```python
from build123d import *

# Parameters (mm, degrees)
SKETCH2_R            = 13.125
F_26_25_MM_HUL_DEPTH = 50
CUT_EXTRUDE1_DEPTH   = 50


with BuildPart() as part:
    # Sketch1 → Base-Revolve (revolve)
    with BuildSketch(Plane.XY):
        with BuildLine():
            Line((28, 0), (28, 39.6))
            ThreePointArc((28, 39.6), (27.882842712, 39.882842712), (27.6, 40))
            Line((27.6, 40), (-74.690598923, 40))
            Line((-74.690598923, 40), (-77, 36))
            Line((-77, 36), (-80, 36))
            Line((-80, 36), (-80, 34.9))
            ThreePointArc((-80, 34.9), (-80.191000574, 34.558943934), (-80.5815962, 34.54359739))
            Line((-80.5815962, 34.54359739), (-81.477336756, 35))
            Line((-81.477336756, 35), (-83.6, 35))
            ThreePointArc((-83.6, 35), (-83.882842712, 34.882842712), (-84, 34.6))
            Line((-84, 34.6), (-84, 25))
            Line((-84, 25), (-47, 25))
            Line((-47, 25), (-32.56624327, 0))
            Line((-32.56624327, 0), (28, 0))
        make_face()
    revolve(axis=Axis((-90.573458716, 0, 0), (1, 0, 0)))

    # Sketch2 → ø26.25 mm hul (cut, symmetric)
    with BuildSketch(Plane.XY):
        Circle(SKETCH2_R)
    extrude(amount=F_26_25_MM_HUL_DEPTH, both=True, mode=Mode.SUBTRACT)

    # Sketch3 → Cut-Extrude1 (cut, symmetric)
    with BuildSketch(Plane(origin=(0, 0, 0), x_dir=(1, 0, 0), z_dir=(0, 1, 0))):
        with BuildLine():
            Line((28, 25), (-39, 25))
            ThreePointArc((-39, 25), (-39.707106781, 25.292893219), (-40, 26))
            Line((-40, 26), (-40, 40))
            Line((-40, 40), (28, 40))
            Line((28, 40), (28, 25))
        make_face()
        with BuildLine():
            Line((-40, -26), (-40, -40))
            Line((-40, -40), (28, -40))
            Line((28, -40), (28, -25))
            Line((28, -25), (-39, -25))
            ThreePointArc((-39, -25), (-39.707106781, -25.292893219), (-40, -26))
        make_face()
    extrude(amount=CUT_EXTRUDE1_DEPTH, both=True, mode=Mode.SUBTRACT)

    # Sketch4 → Cut-Revolve1 (revolve, cut)
    with BuildSketch(Plane.XY):
        Polygon((28, -9.5), (27, -9.5), (27, -14), (8, -14), (6.267949192, -17), (-52, -17), (-55.75277675, -23.5), (28, -23.5), align=None)
    revolve(axis=Axis((28, -23.5, 0), (-1, 0, 0)), mode=Mode.SUBTRACT)


solid = part.part
```
Geometry check sheet. Reference: the model listing, model coordinates, mm. A direction names the side the tool comes from. Give positions to 0.01 mm unless a question says otherwise; leave off trailing zeros. Order: outer loops, then holes, each group sorted by start corner. A loop starts at its lowest first (then second) coordinate and runs counter-clockwise, first axis right, second up. Notation, with made-up numbers: (0, 20) - (15, 20) arc R12 ccw to (15, 31) - close; hole circle Ø6 at (-11.5, -27.75). An arc over 180 degrees is marked (long way). Write item = value, one per line. Start each with the question number.
1) Section check D-D (x = 17). Enter the section's corners in (y, z).
2) Gauge pin test, flat ends, axial feed: pin 1 Ø17 at (y, z) = (-23.5, 0) entering from +X; pin 2 Ø5 at (x, y) = (3.5, -12) entering from -Z; pin 3 Ø10 at (x, z) = (-7, 27.5) entering from -Y. Record the tip position at first contact, or that the pin passes through.
3) Access from +Z, -Z, +X, -X, +Y, -Y to the whole of each face (thin tool, end or side, straight path). Record for faces 1 (the flat face through (-12, 7, 25)), 2 (the cylindrical face through (-65.241, 23.846, 7.509)), 3 (the flat face through (28, 9, 0)), 4 (the conical face through (-53.79, -26.9, -0.07)), 5 (the flat face through (-84, 22.9, 10.4)).
4) Section check B-B (x = -23). Enter the section's corners in (y, z).
5) Section check A-A (x = 0). Enter the section's corners in (y, z) (3 decimals), then the cut area to 3 significant figures.
6) Scan lines: L1, parallel to Z at x = 18.25, y = -23.5; L2, parallel to Y at x = -43.5, z = 5.5; L3, parallel to Z at x = 27.5, y = -23.5. Record each from-to range of solid material in increasing order.
7) Draft check along Y on faces 6 (the cylindrical face through (-35.63, 36.95, -15.32)), 7 (the flat face through (-40, 0, -31)), 8 (the conical face through (-34.871, 3.807, 1.199)). Enter one of: released by +Y, released by -Y, zero draft, split by the parting line, or undercut.
8) Section check C-C (x = -36.5). Enter the section's corners in (y, z), then the cut area to 3 significant figures.
Geometry check:
q1.outline = (-31.22, -25) - (31.22, -25) arc R40 ccw to (31.22, 25) - (-31.22, 25) arc R40 ccw to start; hole circle Ø19 at (-23.5, 0)
q2.pin_1 = 7.42
q2.pin_2 = -25
q2.pin_3 = -33.07
q3.face_1 = +Z, +X, +Y, -Y
q3.face_2 = -X
q3.face_3 = +Z, -Z, +X, +Y, -Y
q3.face_4 = +X
q3.face_5 = +Z, -Z, -X, +Y, -Y
q4.outline = (-31.22, -25) - (31.22, -25) arc R40 ccw to (31.22, 25) - (-31.22, 25) arc R40 ccw to start; hole circle Ø13 at (-23.5, 0)
q5.outline = (-31.225, -25) - (-13.125, -25) - (-13.125, 25) - (-31.225, 25) arc R40 ccw to start; (13.125, -25) - (31.225, -25) arc R40 ccw to (31.225, 25) - (13.125, 25) - close; hole circle Ø13 at (-23.5, 0)
q5.area = 2,280 mm2
q6.L1 = -25 to -9.5, 9.5 to 25
q6.L2 = -39.62 to -26.96, -20.04 to -18.12, 18.12 to 39.62
q6.L3 = -25 to -14, 14 to 25
q7.face_6 = split by the parting line
q7.face_7 = zero draft
q7.face_8 = undercut
q8.outline = (-31.22, -25) - (31.22, -25) arc R40 ccw to (31.22, 25) - (-31.22, 25) arc R40 ccw to start; hole circle Ø13 at (-23.5, 0); hole circle Ø13.63 at (0, 0)
q8.area = 3,440 mm2
